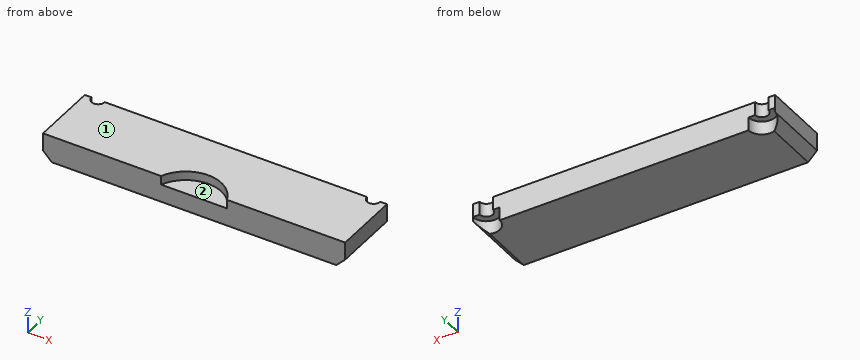
from build123d import *

# Parameters (mm, degrees)
CYLINDER2097_R               = 1.5
CYLINDER2097_DEPTH           = 50
CYLINDER2097_PLACEMENT_ANGLE = 45
CYLINDER2083_R               = 1.5
CYLINDER2083_DEPTH           = 50
CYLINDER2083_PLACEMENT_ANGLE = 45
CYLINDER2096_R               = 1.5
CYLINDER2096_DEPTH           = 50
CYLINDER2096_PLACEMENT_ANGLE = 45
CYLINDER2092_R               = 1.5
CYLINDER2092_DEPTH           = 50
CYLINDER2092_PLACEMENT_ANGLE = 45
CYLINDER2095_R               = 1.5
CYLINDER2095_DEPTH           = 50
CYLINDER2095_PLACEMENT_ANGLE = 45
CYLINDER2094_R               = 1.5
CYLINDER2094_DEPTH           = 50
CYLINDER2094_PLACEMENT_ANGLE = 45
CYLINDER2076_R               = 3
CYLINDER2076_DEPTH           = 3
CYLINDER2076_PLACEMENT_ANGLE = 45
CYLINDER2065_R               = 3
CYLINDER2065_DEPTH           = 3
CYLINDER2065_PLACEMENT_ANGLE = 45
CYLINDER2074_R               = 3
CYLINDER2074_DEPTH           = 3
CYLINDER2074_PLACEMENT_ANGLE = 45
CYLINDER2064_R               = 3
CYLINDER2064_DEPTH           = 3
CYLINDER2064_PLACEMENT_ANGLE = 45
CYLINDER2063_R               = 3
CYLINDER2063_DEPTH           = 3
CYLINDER2063_PLACEMENT_ANGLE = 45
CYLINDER2070_R               = 3
CYLINDER2070_DEPTH           = 3
CYLINDER2070_PLACEMENT_ANGLE = 45
CYLINDER2071_R               = 8
CYLINDER2071_DEPTH           = 6
BOX989_W                     = 68
BOX989_H                     = 15
BOX989_DEPTH                 = 6
CHAMFER081_SIZE              = 2


with BuildPart() as obj1:
    # Cylinder2097 → Cylinder2097 (new body)
    with BuildSketch(Plane.XY):
        Circle(CYLINDER2097_R)
    extrude(amount=CYLINDER2097_DEPTH)


with BuildPart() as obj1_1:
    # Cylinder2097 placement: moved
    add(obj1.part.moved(Location((20, 137, 0))).rotate(Axis((20, 137, 0), (0, 0, 1)), CYLINDER2097_PLACEMENT_ANGLE))


with BuildPart() as compound1087:
    # Cylinder2083 → Cylinder2083 (new body)
    with BuildSketch(Plane.XY):
        Circle(CYLINDER2083_R)
    extrude(amount=CYLINDER2083_DEPTH)


with BuildPart() as compound1087_1:
    # Cylinder2083 placement: moved
    add(compound1087.part.moved(Location((-20, 137, 0))).rotate(Axis((-20, 137, 0), (0, 0, 1)), CYLINDER2083_PLACEMENT_ANGLE))

    # Compound1087: union obj1
    add(obj1_1.part)


with BuildPart() as obj2:
    # Cylinder2096 → Cylinder2096 (new body)
    with BuildSketch(Plane.XY):
        Circle(CYLINDER2096_R)
    extrude(amount=CYLINDER2096_DEPTH)


with BuildPart() as obj2_1:
    # Cylinder2096 placement: moved
    add(obj2.part.moved(Location((31, 131, 0))).rotate(Axis((31, 131, 0), (0, 0, 1)), CYLINDER2096_PLACEMENT_ANGLE))


with BuildPart() as compound1088:
    # Cylinder2092 → Cylinder2092 (new body)
    with BuildSketch(Plane.XY):
        Circle(CYLINDER2092_R)
    extrude(amount=CYLINDER2092_DEPTH)


with BuildPart() as compound1088_1:
    # Cylinder2092 placement: moved
    add(compound1088.part.moved(Location((-31, 131, 0))).rotate(Axis((-31, 131, 0), (0, 0, 1)), CYLINDER2092_PLACEMENT_ANGLE))

    # Compound1088: union obj2
    add(obj2_1.part)


with BuildPart() as obj3:
    # Cylinder2095 → Cylinder2095 (new body)
    with BuildSketch(Plane.XY):
        Circle(CYLINDER2095_R)
    extrude(amount=CYLINDER2095_DEPTH)


with BuildPart() as obj3_1:
    # Cylinder2095 placement: moved
    add(obj3.part.moved(Location((31, 101, 0))).rotate(Axis((31, 101, 0), (0, 0, 1)), CYLINDER2095_PLACEMENT_ANGLE))


with BuildPart() as compound1110:
    # Cylinder2094 → Cylinder2094 (new body)
    with BuildSketch(Plane.XY):
        Circle(CYLINDER2094_R)
    extrude(amount=CYLINDER2094_DEPTH)


with BuildPart() as compound1110_1:
    # Cylinder2094 placement: moved
    add(compound1110.part.moved(Location((-31, 101, 0))).rotate(Axis((-31, 101, 0), (0, 0, 1)), CYLINDER2094_PLACEMENT_ANGLE))

    # Compound1112: union obj3
    add(obj3_1.part)

    # Compound1110: union Compound1087, Compound1088
    add(compound1087_1.part)
    add(compound1088_1.part)


with BuildPart() as obj4:
    # Cylinder2076 → Cylinder2076 (new body)
    with BuildSketch(Plane.XY):
        Circle(CYLINDER2076_R)
    extrude(amount=CYLINDER2076_DEPTH)


with BuildPart() as obj4_1:
    # Cylinder2076 placement: moved
    add(obj4.part.moved(Location((31, 131, 0))).rotate(Axis((31, 131, 0), (0, 0, 1)), CYLINDER2076_PLACEMENT_ANGLE))


with BuildPart() as compound1099:
    # Cylinder2065 → Cylinder2065 (new body)
    with BuildSketch(Plane.XY):
        Circle(CYLINDER2065_R)
    extrude(amount=CYLINDER2065_DEPTH)


with BuildPart() as compound1099_1:
    # Cylinder2065 placement: moved
    add(compound1099.part.moved(Location((-31, 131, 0))).rotate(Axis((-31, 131, 0), (0, 0, 1)), CYLINDER2065_PLACEMENT_ANGLE))

    # Compound1099: union obj4
    add(obj4_1.part)


with BuildPart() as compound1099_2:
    # Compound1099 placement: moved
    add(compound1099_1.part.moved(Location((0, 0, 25))))


with BuildPart() as obj5:
    # Cylinder2074 → Cylinder2074 (new body)
    with BuildSketch(Plane.XY):
        Circle(CYLINDER2074_R)
    extrude(amount=CYLINDER2074_DEPTH)


with BuildPart() as obj5_1:
    # Cylinder2074 placement: moved
    add(obj5.part.moved(Location((31, 101, 0))).rotate(Axis((31, 101, 0), (0, 0, 1)), CYLINDER2074_PLACEMENT_ANGLE))


with BuildPart() as compound1091:
    # Cylinder2064 → Cylinder2064 (new body)
    with BuildSketch(Plane.XY):
        Circle(CYLINDER2064_R)
    extrude(amount=CYLINDER2064_DEPTH)


with BuildPart() as compound1091_1:
    # Cylinder2064 placement: moved
    add(compound1091.part.moved(Location((-31, 101, 0))).rotate(Axis((-31, 101, 0), (0, 0, 1)), CYLINDER2064_PLACEMENT_ANGLE))

    # Compound1091: union obj5
    add(obj5_1.part)


with BuildPart() as compound1091_2:
    # Compound1091 placement: moved
    add(compound1091_1.part.moved(Location((0, 0, 21))))


with BuildPart() as obj6:
    # Cylinder2063 → Cylinder2063 (new body)
    with BuildSketch(Plane.XY):
        Circle(CYLINDER2063_R)
    extrude(amount=CYLINDER2063_DEPTH)


with BuildPart() as obj6_1:
    # Cylinder2063 placement: moved
    add(obj6.part.moved(Location((20, 137, 0))).rotate(Axis((20, 137, 0), (0, 0, 1)), CYLINDER2063_PLACEMENT_ANGLE))


with BuildPart() as compound1096:
    # Cylinder2070 → Cylinder2070 (new body)
    with BuildSketch(Plane.XY):
        Circle(CYLINDER2070_R)
    extrude(amount=CYLINDER2070_DEPTH)


with BuildPart() as compound1096_1:
    # Cylinder2070 placement: moved
    add(compound1096.part.moved(Location((-20, 137, 0))).rotate(Axis((-20, 137, 0), (0, 0, 1)), CYLINDER2070_PLACEMENT_ANGLE))

    # Compound1097: union obj6
    add(obj6_1.part)


with BuildPart() as compound1096_2:
    # Compound1097 placement: moved
    add(compound1096_1.part.moved(Location((0, 0, 25))))

    # Compound1096: union Compound1099, Compound1091
    add(compound1099_2.part)
    add(compound1091_2.part)


with BuildPart() as obj7:
    # Cylinder2071 → Cylinder2071 (new body)
    with BuildSketch(Plane(origin=(0, 83, 25), x_dir=(1, 0, 0), z_dir=(0, 0, 1))):
        Circle(CYLINDER2071_R)
    extrude(amount=CYLINDER2071_DEPTH)


with BuildPart() as cut690:
    # Box989 → Box989 (new body)
    with BuildSketch(Plane(origin=(-34, 86, 21), x_dir=(1, 0, 0), z_dir=(0, 0, 1))):
        with Locations((34, 7.5)):
            Rectangle(BOX989_W, BOX989_H)
    extrude(amount=BOX989_DEPTH)

    # Cut702: cut obj7
    add(obj7.part, mode=Mode.SUBTRACT)

    # Cut700: cut Compound1096
    add(compound1096_2.part, mode=Mode.SUBTRACT)

    # Chamfer081
    chamfer081_edges = [cut690.edges().sort_by_distance(p)[0] for p in [
        (-34, 93.5, 21),
        (34, 93.5, 21),
    ]]
    chamfer(chamfer081_edges, length=CHAMFER081_SIZE)

    # Cut690: cut Compound1110
    add(compound1110_1.part, mode=Mode.SUBTRACT)


solid = cut690.part
Read the model definition and answer for the solid it produces. Units are mm, in the model's axes. Face numbers are marked on the shaded views. Coordinates: 2 decimals unless noted, no trailing zeros. Write each loop counter-clockwise with the first axis right and the second up, starting at its lowest first coordinate (ties: lowest second). Pieces come first, ordered by that corner, then holes. Notation, with made-up numbers: M 35,49 L 69,49 A30 cw 69,72 Z; hole C -21,58.5 d1. An arc over 180 degrees is marked long. Use a Markdown table: item, result.
Q1. Straight lines are drawn through the part: L1, parallel to X at y = 99.25, z = 22.8; L2, parallel to Z at x = 30.5, y = 99.5; L3, parallel to Z at x = 0, y = 88. For each, find the intervals that lie inside material, in ascending order. Write a range as [from, to].
Answer block:
| item | result |
|---|---|
| L1 | x = [-33.8, -33.44], [-28.56, 28.56], [33.44, 33.8] |
| L2 | z = [24, 27] |
| L3 | z = [21, 25] |
Q2. The part is cut by section B-B, the plane y = 89.75. Write down the section's boundary in (x, z), then the cut area to 3 significant figures.
Answer block:
| item | result |
|---|---|
| outline | M -34,23 L -32,21 L 32,21 L 34,23 L 34,27 L 4.29,27 L 4.29,25 L -4.29,25 L -4.29,27 L -34,27 Z |
| area | 387 mm2 |
Q3. Determine the mould class of the marked faces 1 and 2 for opening direction X: released by +X, released by -X, zero draft, split by the parting line, or undercut.
Answer block:
| item | result |
|---|---|
| face 1 | zero draft |
| face 2 | undercut |
Q4. Each of these flat-tipped pins is pushed along its axis until it touches: pin 1 Ø1.5 at (x, y) = (-30.5, 100) entering from -Z; pin 2 Ø3.5 at (x, y) = (32.5, 99.5) entering from -Z. Where does it stop, or does it pass through?
Answer block:
| item | result |
|---|---|
| pin 1 | stops at z = 24 |
| pin 2 | stops at z = 21 |
Q5. The part is cut by section C-C, the plane z = 21.85. Write down the section's boundary in (x, y).
Answer block:
| item | result |
|---|---|
| outline | M -32.85,86 L 32.85,86 L 32.85,98.64 A3 cw 28,101 L -28,101 A3 cw -32.85,98.64 Z |
Q6. The part is cut by section A-A, the plane x = -31. Write down the section's boundary in (y, z), then the cut area to 3 significant figures.
Answer block:
| item | result |
|---|---|
| outline | M 86,21 L 98,21 L 98,24 L 99.5,24 L 99.5,27 L 86,27 Z |
| area | 76.5 mm2 |
